```python
from build123d import *

# Parameters (mm, degrees)
SKETCH2_W           = 220
SKETCH2_H           = 220
BOSS_EXTRUDE1_DEPTH = 6
SKETCH3_R           = 13.5
CUT_EXTRUDE1_DEPTH  = 10
SKETCH4_R           = 2.5
CUT_EXTRUDE2_DEPTH  = 10
CAVITY1_START       = -197.339948834
CAVITY1_OUTLINE_W   = 6
CAVITY1_OUTLINE_H   = 6
CAVITY1_DEPTH       = 15
CAVITY1_START_2     = -142.339948834
CAVITY1_2_OUTLINE_W = 6
CAVITY1_2_OUTLINE_H = 6
CAVITY1_2_DEPTH     = 15
CAVITY1_START_3     = -77.339948834
CAVITY1_3_OUTLINE_W = 6
CAVITY1_3_OUTLINE_H = 6
CAVITY1_3_DEPTH     = 15
CAVITY1_START_4     = -22.339948834
CAVITY1_4_OUTLINE_W = 6
CAVITY1_4_OUTLINE_H = 6
CAVITY1_4_DEPTH     = 15
CAVITY1_START_5     = -212.339948834
CAVITY1_5_OUTLINE_W = 15
CAVITY1_5_OUTLINE_H = 6
CAVITY1_5_DEPTH     = 6
CAVITY1_START_6     = 1.660051166
CAVITY1_6_OUTLINE_W = 15
CAVITY1_6_OUTLINE_H = 6
CAVITY1_6_DEPTH     = 6
SKETCH5_W           = 6.5
SKETCH5_H           = 16
SKETCH5_W_2         = 7
SKETCH5_W_3         = 16
SKETCH5_H_2         = 6.5
CUT_EXTRUDE3_DEPTH  = 10


# Read off the part's stored shape, not the designer's step: Cavity1
with BuildPart() as part:
    # Sketch2 → Boss-Extrude1 (new body)
    with BuildSketch(Plane(origin=(0, 0, 0), x_dir=(1, 0, 0), z_dir=(0, 1, 0))):
        with Locations((-604.222894392, 102.339948834)):
            Rectangle(SKETCH2_W, SKETCH2_H)
    extrude(amount=BOSS_EXTRUDE1_DEPTH)

    # Sketch3 → Cut-Extrude1 (cut)
    with BuildSketch(Plane(origin=(0, 6, 0), x_dir=(1, 0, 0), z_dir=(0, 1, 0))):
        with Locations(Location((-616.722894392, 102.339948834, 0), (0, 0, 270))):
            Circle(SKETCH3_R)
    extrude(amount=-CUT_EXTRUDE1_DEPTH, mode=Mode.SUBTRACT)

    # Sketch4 → Cut-Extrude2 (cut)
    with BuildSketch(Plane(origin=(0, 6, 0), x_dir=(1, 0, 0), z_dir=(0, 1, 0))):
        with Locations(Location((-590.222894392, 102.339948834, 0), (0, 0, 270))):
            Circle(SKETCH4_R)
        with Locations(Location((-616.722894392, 128.839948834, 0), (0, 0, 270))):
            Circle(SKETCH4_R)
        with Locations(Location((-643.222894392, 102.339948834, 0), (0, 0, 270))):
            Circle(SKETCH4_R)
        with Locations(Location((-616.722894392, 75.839948834, 0), (0, 0, 270))):
            Circle(SKETCH4_R)
    extrude(amount=-CUT_EXTRUDE2_DEPTH, mode=Mode.SUBTRACT)

    # Cavity1 outline → Cavity1 (cut)
    with BuildSketch(Plane.XY.offset(CAVITY1_START)):
        with Locations((-633.222894392, 3)):
            Rectangle(CAVITY1_OUTLINE_W, CAVITY1_OUTLINE_H)
        with Locations((-600.222894392, 3)):
            Rectangle(CAVITY1_OUTLINE_W, CAVITY1_OUTLINE_H)
        with Locations((-497.222894392, 3)):
            Rectangle(CAVITY1_OUTLINE_W, CAVITY1_OUTLINE_H)
    extrude(amount=CAVITY1_DEPTH, mode=Mode.SUBTRACT)

    # Cavity1 2 outline → Cavity1 2 (cut)
    with BuildSketch(Plane.XY.offset(CAVITY1_START_2)):
        with Locations((-633.222894392, 3)):
            Rectangle(CAVITY1_2_OUTLINE_W, CAVITY1_2_OUTLINE_H)
        with Locations((-600.222894392, 3)):
            Rectangle(CAVITY1_2_OUTLINE_W, CAVITY1_2_OUTLINE_H)
        with Locations((-497.222894392, 3)):
            Rectangle(CAVITY1_2_OUTLINE_W, CAVITY1_2_OUTLINE_H)
    extrude(amount=CAVITY1_2_DEPTH, mode=Mode.SUBTRACT)

    # Cavity1 3 outline → Cavity1 3 (cut)
    with BuildSketch(Plane.XY.offset(CAVITY1_START_3)):
        with Locations((-633.222894392, 3)):
            Rectangle(CAVITY1_3_OUTLINE_W, CAVITY1_3_OUTLINE_H)
        with Locations((-600.222894392, 3)):
            Rectangle(CAVITY1_3_OUTLINE_W, CAVITY1_3_OUTLINE_H)
        with Locations((-497.222894392, 3)):
            Rectangle(CAVITY1_3_OUTLINE_W, CAVITY1_3_OUTLINE_H)
    extrude(amount=CAVITY1_3_DEPTH, mode=Mode.SUBTRACT)

    # Cavity1 4 outline → Cavity1 4 (cut)
    with BuildSketch(Plane.XY.offset(CAVITY1_START_4)):
        with Locations((-633.222894392, 3)):
            Rectangle(CAVITY1_4_OUTLINE_W, CAVITY1_4_OUTLINE_H)
        with Locations((-600.222894392, 3)):
            Rectangle(CAVITY1_4_OUTLINE_W, CAVITY1_4_OUTLINE_H)
        with Locations((-497.222894392, 3)):
            Rectangle(CAVITY1_4_OUTLINE_W, CAVITY1_4_OUTLINE_H)
    extrude(amount=CAVITY1_4_DEPTH, mode=Mode.SUBTRACT)

    # Cavity1 5 outline → Cavity1 5 (cut)
    with BuildSketch(Plane.XY.offset(CAVITY1_START_5)):
        with Locations((-653.722894392, 3)):
            Rectangle(CAVITY1_5_OUTLINE_W, CAVITY1_5_OUTLINE_H)
        with Locations((-696.722894392, 3)):
            Rectangle(CAVITY1_5_OUTLINE_W, CAVITY1_5_OUTLINE_H)
    extrude(amount=CAVITY1_5_DEPTH, mode=Mode.SUBTRACT)

    # Cavity1 6 outline → Cavity1 6 (cut)
    with BuildSketch(Plane.XY.offset(CAVITY1_START_6)):
        with Locations((-653.722894392, 3)):
            Rectangle(CAVITY1_6_OUTLINE_W, CAVITY1_6_OUTLINE_H)
        with Locations((-696.722894392, 3)):
            Rectangle(CAVITY1_6_OUTLINE_W, CAVITY1_6_OUTLINE_H)
    extrude(amount=CAVITY1_6_DEPTH, mode=Mode.SUBTRACT)

    # Sketch5 → Cut-Extrude3 (cut)
    with BuildSketch(Plane(origin=(0, 6, 0), x_dir=(1, 0, 0), z_dir=(0, 1, 0))):
        with Locations((-497.472894392, 14.839948834)):
            Rectangle(SKETCH5_W, SKETCH5_H)
        with Locations((-497.472894392, 69.839948834)):
            Rectangle(SKETCH5_W, SKETCH5_H)
        with Locations((-497.472894392, 134.839948834)):
            Rectangle(SKETCH5_W, SKETCH5_H)
        with Locations((-497.472894392, 189.839948834)):
            Rectangle(SKETCH5_W, SKETCH5_H)
        with Locations((-600.222894392, 189.839948834)):
            Rectangle(SKETCH5_W_2, SKETCH5_H)
        with Locations((-633.222894392, 189.839948834)):
            Rectangle(SKETCH5_W_2, SKETCH5_H)
        with Locations((-600.222894392, 134.839948834)):
            Rectangle(SKETCH5_W_2, SKETCH5_H)
        with Locations((-600.222894392, 69.839948834)):
            Rectangle(SKETCH5_W_2, SKETCH5_H)
        with Locations((-600.222894392, 14.839948834)):
            Rectangle(SKETCH5_W_2, SKETCH5_H)
        with Locations((-633.222894392, 134.839948834)):
            Rectangle(SKETCH5_W_2, SKETCH5_H)
        with Locations((-633.222894392, 69.839948834)):
            Rectangle(SKETCH5_W_2, SKETCH5_H)
        with Locations((-633.222894392, 14.839948834)):
            Rectangle(SKETCH5_W_2, SKETCH5_H)
        with Locations((-653.722894392, 209.089948834)):
            Rectangle(SKETCH5_W_3, SKETCH5_H_2)
        with Locations((-696.722894392, 209.089948834)):
            Rectangle(SKETCH5_W_3, SKETCH5_H_2)
        with Locations((-653.722894392, -4.410051166)):
            Rectangle(SKETCH5_W_3, SKETCH5_H_2)
        with Locations((-696.722894392, -4.410051166)):
            Rectangle(SKETCH5_W_3, SKETCH5_H_2)
    extrude(amount=-CUT_EXTRUDE3_DEPTH, mode=Mode.SUBTRACT)


solid = part.part
```
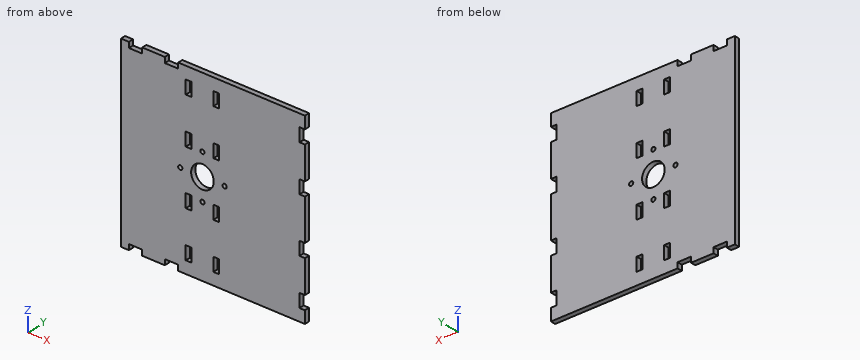
Work out the finished part from the listing and answer in its coordinate system (mm). Give positions to 0.01 mm unless a question says otherwise; leave off trailing zeros. Write each loop counter-clockwise with the first axis right and the second up, starting at its lowest first coordinate (ties: lowest second). Pieces come first, ordered by that corner, then holes. Notation, with made-up numbers: (-13.5, -40) -> (8.5, -40) arc R12 ccw to (8.5, -23) -> close; hole circle Ø9 at (-30, 59.25). An arc over 180 degrees is marked (long way). Write each question's results on one line, items separated by ' | '.
1. Straight lines are drawn through the part: L1, parallel to X at y = 2.6, z = -64.5; L2, parallel to Z at x = -635, y = 5.8; L3, parallel to Z at x = -619.5, y = 4.35. For each, find the intervals that lie inside material, in ascending order.
Data:
L1: -714.22 to -636.72, -629.72 to -603.72, -596.72 to -500.72 | L2: -212.34 to -197.84, -181.84 to -142.84, -126.84 to -77.84, -61.84 to -22.84, -6.84 to 7.66 | L3: -212.34 to -115.55, -89.13 to 7.66
2. Find section A-A on z = -64.5. Determine the outline of the cut face in (x, y), and give its area (3 significant figures).
Data:
outline: (-714.22, 0) -> (-636.72, 0) -> (-636.72, 6) -> (-714.22, 6) -> close; (-629.72, 0) -> (-603.72, 0) -> (-603.72, 6) -> (-629.72, 6) -> close; (-596.72, 0) -> (-500.72, 0) -> (-500.72, 6) -> (-596.72, 6) -> close | area: 1,200 mm^2
3. Find section C-C on x = -692.5. Determine the outline of the cut face in (y, z).
Data:
outline: (0, -205.84) -> (6, -205.84) -> (6, 1.16) -> (0, 1.16) -> close
4. Each of these flat-tipped pins is pushed along its axis until it touches: pin 1 Ø2 at (y, z) = (3, -76.5) entering from +X; pin 2 Ø8 at (x, z) = (-616.72, -128.84) entering from -Y. Where does it stop, or does it pass through?
Data:
pin 1: x = -500.72 | pin 2: y = 0
5. Find section D-D on y = 4.75. Give the number of separate pieces and of enclosed holes in the cut face, and give its area (3 significant figures).
Data:
separate pieces: 1 | enclosed holes: 13 | area: 46,000 mm^2
6. Find section B-B on z = -109. Determine the outline of the cut face in (x, y).
Data:
outline: (-714.22, 0) -> (-628.47, 0) -> (-628.47, 6) -> (-714.22, 6) -> close; (-604.98, 0) -> (-494.22, 0) -> (-494.22, 6) -> (-604.98, 6) -> close
